Can you work these out from the drawing? Everything is in mm from the part's minimum corner. A direction names the side the tool comes from. Coordinates: 2 decimals unless noted, no trailing zeros. Order: outer loops, then holes, each group sorted by start corner. A loop starts at its lowest first (then second) coordinate and runs counter-clockwise, first axis right, second up. Notation, with made-up numbers: (10.5, -34) -> (40.5, -34) arc R22 ccw to (40.5, -12) -> close; hole circle Ø4 at (-18.5, -4). An arc over 180 degrees is marked (long way). Put each result on its own line as item: value. Start each with the question number.
Q1. If we section it at A-A (y = 12): Please give me the cut outline in (x, z).
Q2. Please list where these lines run through material, in increasing order: line 1 along Y through (x, z) = (0.75, 27.5); line 2 along X through (y, z) = (76, 20.5); line 3 along Z through (x, y) = (21.75, 33).
Q3. For the marked faces 1 and 2, which set-ups out of +Z, -Z, +X, -X, +Y, -Y let a thin tool reach every point of the face, with its end or its side?
Q4. We'd pull the mould along Z, two halves only. Please class the marked faces 3, 4 and 5: +Z half, -Z half, draft (parallel to the pull), parting line (faces both ways), or undercut.
Q5. If we section it at C-C (z = 31): Please give me the cut outline in (x, y).
Q6. If we section it at D-D (z = 13): Please give me the cut outline in (x, y).
Q7. If we section it at B-B (x = 7.5): Please give me the cut outline in (y, z).
Q8. Will this pin go through, and if not, where does the flat tip stop? pin 1 (1.9 mm diameter, centred on y = 62, z = 12.5, fed in from -X).
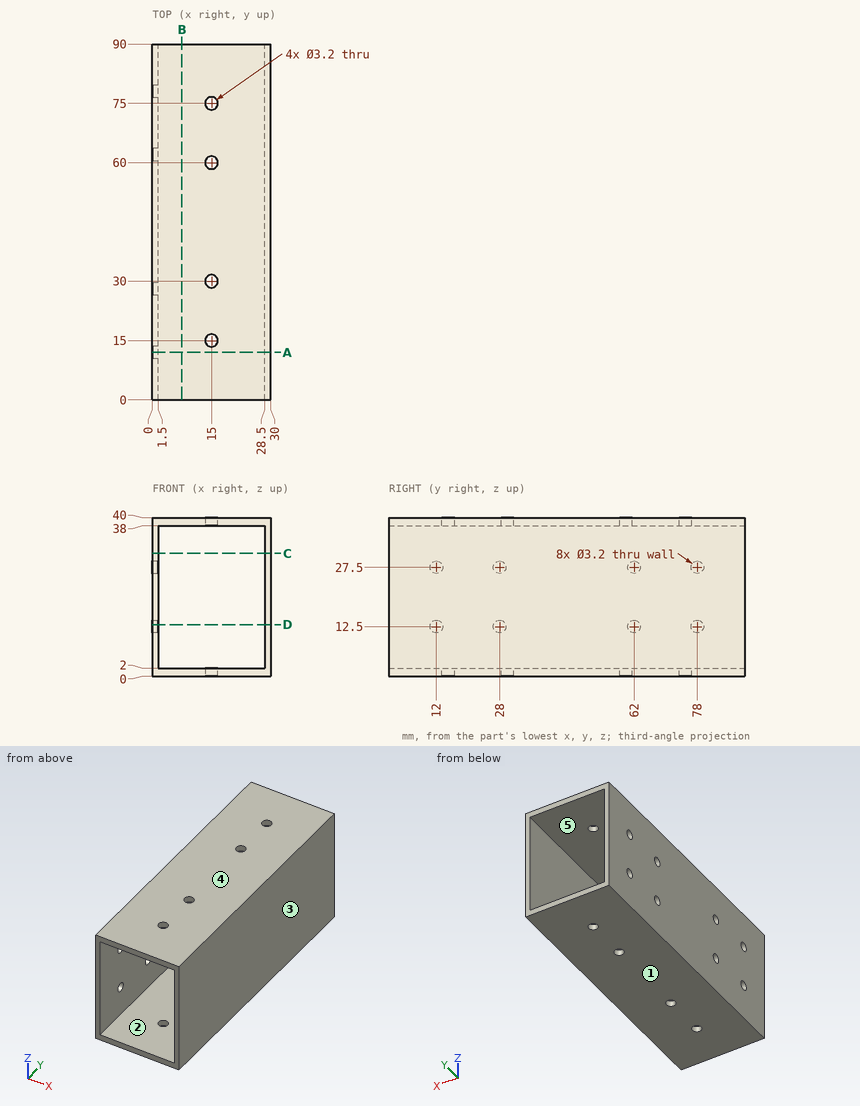
The answers:
1. outline: (0, 0) -> (30, 0) -> (30, 40) -> (0, 40) -> (0, 29.1) -> (1.5, 29.1) -> (1.5, 38) -> (28.5, 38) -> (28.5, 2) -> (1.5, 2) -> (1.5, 10.9) -> (0, 10.9) -> close; (0, 14.1) -> (1.5, 14.1) -> (1.5, 25.9) -> (0, 25.9) -> close
2. line 1: 0 to 10.4, 13.6 to 26.4, 29.6 to 60.4, 63.6 to 76.4, 79.6 to 90
2. line 2: 0 to 1.5, 28.5 to 30
2. line 3: 0 to 2, 38 to 40
3. face 1: -Z, +X, -X, +Y, -Y
3. face 2: +Y, -Y
4. face 3: draft
4. face 4: +Z half
4. face 5: undercut
5. outline: (0, 0) -> (1.5, 0) -> (1.5, 90) -> (0, 90) -> close; (28.5, 0) -> (30, 0) -> (30, 90) -> (28.5, 90) -> close
6. outline: (0, 0) -> (1.5, 0) -> (1.5, 10.48) -> (0, 10.48) -> close; (0, 13.52) -> (1.5, 13.52) -> (1.5, 26.48) -> (0, 26.48) -> close; (0, 29.52) -> (1.5, 29.52) -> (1.5, 60.48) -> (0, 60.48) -> close; (0, 63.52) -> (1.5, 63.52) -> (1.5, 76.48) -> (0, 76.48) -> close; (0, 79.52) -> (1.5, 79.52) -> (1.5, 90) -> (0, 90) -> close; (28.5, 0) -> (30, 0) -> (30, 90) -> (28.5, 90) -> close
7. outline: (0, 0) -> (90, 0) -> (90, 2) -> (0, 2) -> close; (0, 38) -> (90, 38) -> (90, 40) -> (0, 40) -> close
8. pin 1: x = 28.5
